Here's how the part is built. I have some questions about the finished solid (model axes, mm). Face numbers are marked on the shaded views. A direction names the side the tool comes from. Give positions to 0.01 mm unless a question says otherwise; leave off trailing zeros. Write each loop counter-clockwise with the first axis right and the second up, starting at its lowest first coordinate (ties: lowest second). Pieces come first, ordered by that corner, then holes. Notation, with made-up numbers: M 66.25,57.5 L 91.25,57.5 A15 ccw 91.25,71.5 Z; hole C 69.25,26 d11. An arc over 180 degrees is marked long. Answer as CSV lines item,"result". Start each with the question number.
Q1. Suppose I cut it at A-A (y = 10.5). Write out the boundary of the cut face in (x, z).
Q2. Suppose I cut it at B-B (x = -7). Write out the boundary of the cut face in (y, z), then the cut area to 3 significant figures.
Q3. On a 3-axis mill with a long thin cutter (end or side, diameter ignored), from which of +Z, -Z, +X, -X, +Y, -Y can I reach the whole of each face in a straight line? I mean the marked faces 5, 6, 7, 8 and 9. Say none if no direction works.
Q4. For pin 1 (5 mm diameter, centred on x = 11, z = 8, fed in from +Y); pin 2 (3.5 mm diameter, centred on x = -10.5, z = 5, fed in from +Y); pin 3 (9 mm diameter, centred on x = -1.5, y = 2.5, fed in from +Z); pin 4 (5 mm diameter, centred on x = -12.5, z = 5.5, fed in from -Y), each with a flat end and sliding along its axis, tell me the tip position at first contact or that it passes through.
Q5. If I drill on line 1 along Y through (x, z) = (9.5, 11); line 2 along Y through (x, z) = (7, 2.25); line 3 along X through (y, z) = (1, 11.5), over which ranges is the centre line in solid material (lowest first)?
Q6. Thinking about a two-plate mould opening in Y: for the marked faces 1, 2, 3 and 4, which applies, +Y half, -Y half, draft (parallel to the pull), parting line (faces both ways), or undercut?
```python
from build123d import *

# Parameters (mm, degrees)
F1_DEPTH     = 12.7508
F2_START     = 2.3114
F2_DEPTH     = 8.128
F3_R         = 1.27
F4_T4_DEPTH  = 13.1696453782
F4_S5_R      = 3.9624
F4_T6_DEPTH  = 8
F4_T15_DEPTH = 13.1696453782
F4_S16_R     = 3.9624
F4_T17_DEPTH = 8


# Not quite as in the source:
# - a fillet or chamfer that OpenCascade refuses, or shapes differently, is made with other operations: its cross-section is extruded or revolved along the edge and cut away or added
# - a feature names something its author has since deleted; it is built from what else it names


with BuildPart() as f1:
    # F0 (on Top) → F1 (new body)
    with BuildSketch(Plane.XY):
        with BuildLine():
            ThreePointArc((0, -5.7023), (-5.7023, 0), (0, 5.7023))
            Line((0, 5.7023), (0, 8.2296))
            ThreePointArc((0, 8.2296), (-1.596599089, 8.0732389726), (-3.1325279453, 7.6100975573))
            Line((-3.1325279453, 7.6100975573), (-5.9126210852, 12.4253601255))
            ThreePointArc((-5.9126210852, 12.4253601255), (-8.73125, 15.1229686136), (-7.8043669773, 11.3331601255))
            Line((-7.8043669773, 11.3331601255), (-5.0242738373, 6.5178975573))
            ThreePointArc((-5.0242738373, 6.5178975573), (-7.127042663, 4.1148), (-8.1568017826, 1.0922))
            Line((-8.1568017826, 1.0922), (-13.7169880625, 1.0922))
            ThreePointArc((-13.7169880625, 1.0922), (-17.4625, 0), (-13.7169880625, -1.0922))
            Line((-13.7169880625, -1.0922), (-8.1568017826, -1.0922))
            ThreePointArc((-8.1568017826, -1.0922), (-7.127042663, -4.1148), (-5.0242738373, -6.5178975573))
            Line((-5.0242738373, -6.5178975573), (-7.8043669773, -11.3331601255))
            ThreePointArc((-7.8043669773, -11.3331601255), (-8.73125, -15.1229686136), (-5.9126210852, -12.4253601255))
            Line((-5.9126210852, -12.4253601255), (-3.1325279453, -7.6100975573))
            ThreePointArc((-3.1325279453, -7.6100975573), (-1.596599089, -8.0732389726), (0, -8.2296))
            Line((0, -8.2296), (0, -5.7023))
        make_face()
        with BuildLine():
            ThreePointArc((0, 5.7023), (4.0321349984, 4.0321349984), (5.7023, 0))
            ThreePointArc((5.7023, 0), (4.0321349984, -4.0321349984), (0, -5.7023))
            Line((0, -5.7023), (0, -8.2296))
            ThreePointArc((0, -8.2296), (1.596599089, -8.0732389726), (3.1325279453, -7.6100975573))
            Line((3.1325279453, -7.6100975573), (5.9126210852, -12.4253601255))
            ThreePointArc((5.9126210852, -12.4253601255), (8.73125, -15.1229686136), (7.8043669773, -11.3331601255))
            Line((7.8043669773, -11.3331601255), (5.0242738373, -6.5178975573))
            ThreePointArc((5.0242738373, -6.5178975573), (7.127042663, -4.1148), (8.1568017826, -1.0922))
            Line((8.1568017826, -1.0922), (13.7169880625, -1.0922))
            ThreePointArc((13.7169880625, -1.0922), (15.9993443297, -1.9507537334), (17.4625, 0))
            ThreePointArc((17.4625, 0), (15.9993443297, 1.9507537334), (13.7169880625, 1.0922))
            Line((13.7169880625, 1.0922), (8.1568017826, 1.0922))
            ThreePointArc((8.1568017826, 1.0922), (7.127042663, 4.1148), (5.0242738373, 6.5178975573))
            Line((5.0242738373, 6.5178975573), (7.8043669773, 11.3331601255))
            ThreePointArc((7.8043669773, 11.3331601255), (8.73125, 15.1229686136), (5.9126210852, 12.4253601255))
            Line((5.9126210852, 12.4253601255), (3.1325279453, 7.6100975573))
            ThreePointArc((3.1325279453, 7.6100975573), (1.596599089, 8.0732389726), (0, 8.2296))
            Line((0, 8.2296), (0, 5.7023))
        make_face()
    extrude(amount=F1_DEPTH)

    # F0 (on Top) → F2 (join)
    with BuildSketch(Plane.XY.offset(F2_START)):
        with BuildLine():
            Line((0, 3.9624), (0, 5.7023))
            ThreePointArc((0, 5.7023), (-5.7023, 0), (0, -5.7023))
            Line((0, -5.7023), (0, -3.1496))
            Line((0, -3.1496), (-2.4042948239, -3.1496))
            ThreePointArc((-2.4042948239, -3.1496), (-3.7537040906, 1.2689835933), (0, 3.9624))
        make_face()
        with BuildLine():
            ThreePointArc((0, -5.7023), (4.0321349984, -4.0321349984), (5.7023, 0))
            ThreePointArc((5.7023, 0), (4.0321349984, 4.0321349984), (0, 5.7023))
            Line((0, 5.7023), (0, 3.9624))
            ThreePointArc((0, 3.9624), (3.7537040906, 1.2689835933), (2.4042948239, -3.1496))
            Line((2.4042948239, -3.1496), (0, -3.1496))
            Line((0, -3.1496), (0, -5.7023))
        make_face()
    extrude(amount=F2_DEPTH)

    # F3
    f3_edges = [f1.edges().sort_by_distance(p)[0] for p in [
        (-8.156802, 1.0922, 6.3754),
        (-8.156802, -1.0922, 6.3754),
        (3.132528, 7.610098, 6.3754),
        (-3.132528, 7.610098, 6.3754),
        (5.024274, 6.517898, 6.3754),
        (8.156802, 1.0922, 6.3754),
        (8.156802, -1.0922, 6.3754),
        (5.024274, -6.517898, 6.3754),
        (3.132528, -7.610098, 6.3754),
        (-3.132528, -7.610098, 6.3754),
        (-5.024274, -6.517898, 6.3754),
        (-5.024274, 6.517898, 6.3754),
    ]]
    fillet(f3_edges, radius=F3_R)

    # F4: chamfer of 1.6256 on 4 edges, made by hand


with BuildPart() as f4_tool2:
    # F4_s3 → F4_t4 (new body)
    with BuildSketch(Plane.YZ.offset(6.5848226891)):
        Polygon((-3.1496, 3.937), (-4.7752, 2.3114), (-3.1496, 2.3114), align=None)
    extrude(amount=-F4_T4_DEPTH)

    # F4_s5 → F4_t6 (intersect, symmetric)
    with BuildSketch(Plane.XY.offset(3.1)):
        Circle(F4_S5_R)
    extrude(amount=F4_T6_DEPTH, both=True, mode=Mode.INTERSECT)


with BuildPart() as f1_1:
    add(f1.part)

    # F4_t1: cut F4_tool2
    add(f4_tool2.part, mode=Mode.SUBTRACT)


with BuildPart() as f4_tool8:
    # F4_s9 → F4_t10 (revolve)
    with BuildSketch(Plane(origin=(0, 0, 0), x_dir=(0, 0, 1), z_dir=(0.7948717949, -0.6067774137, 0))):
        Polygon((3.937, 3.9624), (2.3114, 5.588), (2.3114, 3.9624), align=None)
    revolve(axis=Axis((0, 0, 2.3114), (0, 0, -1)))

    split(bisect_by=Plane(origin=(0, -3.5433, 3.5433), x_dir=(1, 0, 0), z_dir=(0, 0.7071067812, -0.7071067812)), keep=Keep.TOP)


with BuildPart() as f1_2:
    add(f1_1.part)

    # F4_t7: cut F4_tool8
    add(f4_tool8.part, mode=Mode.SUBTRACT)


with BuildPart() as f4_tool13:
    # F4_s14 → F4_t15 (new body)
    with BuildSketch(Plane.YZ.offset(6.5848226891)):
        Polygon((-4.7752, 10.4394), (-3.1496, 8.8138), (-3.1496, 10.4394), align=None)
    extrude(amount=-F4_T15_DEPTH)

    # F4_s16 → F4_t17 (intersect, symmetric)
    with BuildSketch(Plane.XY.offset(9.6)):
        Circle(F4_S16_R)
    extrude(amount=F4_T17_DEPTH, both=True, mode=Mode.INTERSECT)


with BuildPart() as f1_3:
    add(f1_2.part)

    # F4_t12: cut F4_tool13
    add(f4_tool13.part, mode=Mode.SUBTRACT)


with BuildPart() as f4_tool19:
    # F4_s20 → F4_t21 (revolve)
    with BuildSketch(Plane(origin=(0, 0, 0), x_dir=(0, 0, 1), z_dir=(0.7948717949, -0.6067774137, 0))):
        Polygon((10.4394, 5.588), (8.8138, 3.9624), (10.4394, 3.9624), align=None)
    revolve(axis=Axis((0, 0, 10.4394), (0, 0, -1)))

    split(bisect_by=Plane(origin=(0, 2.8321, 2.8321), x_dir=(1, 0, 0), z_dir=(0, 0.7071067812, 0.7071067812)), keep=Keep.TOP)


with BuildPart() as f1_4:
    add(f1_3.part)

    # F4_t18: cut F4_tool19
    add(f4_tool19.part, mode=Mode.SUBTRACT)


solid = f1_4.part
```
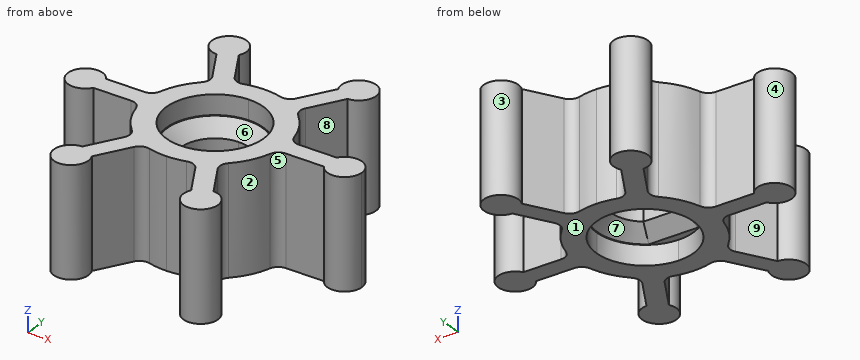
Resolved:
1,outline,"M -7.32,0 L -4.8,0 L -4.8,12.75 L -7.32,12.75 Z; M 4.8,0 L 7.32,0 L 7.32,12.75 L 4.8,12.75 Z"
2,outline,"M -15.27,0 L -9.94,0 L -9.94,12.75 L -15.27,12.75 Z; M -4.33,0 L 4.33,0 L 4.33,12.75 L -4.33,12.75 Z; M 9.94,0 L 15.27,0 L 15.27,12.75 L 9.94,12.75 Z"
2,area,"246 mm^2"
3,face 5,"+Z, -Z"
3,face 6,"+Z"
3,face 7,"-Z"
3,face 8,"+Z, -Z, +X"
3,face 9,"+Z, -Z, -X"
4,pin 1,"y = 15.24"
4,pin 2,"y = 15.11"
4,pin 3,"z = 12.75"
4,pin 4,"y = -1.99"
5,line 1,"-14.33 to -12.39, -1.09 to 1.09, 12.39 to 14.33"
5,line 2,"-15.27 to -9.94, -4.33 to 4.33, 9.94 to 15.27"
5,line 3,"-17.2 to -5.61, 5.61 to 17.2"
6,face 1,"draft"
6,face 2,"undercut"
6,face 3,"undercut"
6,face 4,"parting line"
